from build123d import *

# Parameters (mm, degrees)
F1_DEPTH = 40.2336
F0_R     = 10.16
F2_DEPTH = 15.7734
F3_R     = 3.302


# Not quite as in the source:
# - a feature names something its author has since deleted; it is built from what else it names


with BuildPart() as f1:
    # F0 (on Top) → F1 (new body)
    with BuildSketch(Plane.XY):
        with BuildLine():
            ThreePointArc((-48.9323529412, -28.1265414802), (-32.0589754437, -18.3362616868), (-25.4, 0))
            ThreePointArc((-25.4, 0), (-32.0589754437, 18.3362616868), (-48.9323529412, 28.1265414802))
            ThreePointArc((-48.9323529412, 28.1265414802), (-82.55, 0), (-48.9323529412, -28.1265414802))
        make_face()
        with BuildLine():
            ThreePointArc((-40.5272351207, -4.826), (-68.2625, 0), (-40.5272351207, 4.826))
            Line((-40.5272351207, 4.826), (-34.1772351207, 4.826))
            Line((-34.1772351207, 4.826), (-34.1772351207, -4.826))
            Line((-34.1772351207, -4.826), (-40.5272351207, -4.826))
        make_face(mode=Mode.SUBTRACT)
    extrude(amount=F1_DEPTH)

    # F0 (on Top) → F2 (join)
    with BuildSketch(Plane.XY):
        with BuildLine():
            ThreePointArc((-48.9323529412, 28.1265414802), (-32.0589754437, 18.3362616868), (-25.4, 0))
            ThreePointArc((-25.4, 0), (-32.0589754437, -18.3362616868), (-48.9323529412, -28.1265414802))
            Line((-48.9323529412, -28.1265414802), (3.3617647059, -18.7510276535))
            ThreePointArc((3.3617647059, -18.7510276535), (-19.05, 0), (3.3617647059, 18.7510276535))
            Line((3.3617647059, 18.7510276535), (-48.9323529412, 28.1265414802))
        make_face()
        with BuildLine():
            ThreePointArc((19.05, 0), (14.6106830375, 12.2241744579), (3.3617647059, 18.7510276535))
            ThreePointArc((3.3617647059, 18.7510276535), (-19.05, 0), (3.3617647059, -18.7510276535))
            ThreePointArc((3.3617647059, -18.7510276535), (14.6106830375, -12.2241744579), (19.05, 0))
        make_face()
        Circle(F0_R, mode=Mode.SUBTRACT)
    extrude(amount=F2_DEPTH)

    # F3
    f3_edges = [f1.edges().sort_by_distance(p)[0] for p in [
        (-59.017647, 28.126541, 40.2336),
    ]]
    fillet(f3_edges, radius=F3_R)


solid = f1.part
Geometry: final body of the model. Coordinates: model frame, mm. A direction names the side the tool comes from. Give positions to 0.01 mm unless a question says otherwise; leave off trailing zeros. Order: outer loops, then holes, each group sorted by start corner. A loop starts at its lowest first (then second) coordinate and runs counter-clockwise, first axis right, second up. Notation, with made-up numbers: (67, 35) -> (106, 35) arc R21 ccw to (106, 58) -> close; hole circle Ø3 at (36.5, 1). An arc over 180 degrees is marked (long way). Write each question's results on one line, items separated by ' | '.
1) Draft query along Y for faces 1 (the face through (-22.419, 23.373, 7.776)), 2 (the face through (-37, -4.826, 20)), 3 (the face through (-23.151, -23.504, 7.776)). Return one class per face: released by +Y, released by -Y, zero draft, split by the parting line, or undercut.
Geometry says:
face 1: released by +Y | face 2: undercut | face 3: released by -Y
2) Set-up query: faces 4 (the face through (-32, 0, 0)), 5 (the face through (-37, 4.826, 20)). Return all of +Z, -Z, +X, -X, +Y, -Y with unobstructed straight access to the full face (end or side cutting, diameter ignored); none if empty.
Geometry says:
face 4: -Z, +X, -X, +Y, -Y | face 5: +Z, -Z
3) First-contact query: pin 1 Ø5 at (x, z) = (-38, 14.5) entering from +Y; pin 2 Ø7.5 at (y, z) = (-0.5, 25.5) entering from -X; pin 3 Ø1 at (x, y) = (-20, -6) entering from +Z. Flat tips, straight axial feed; report the tip coordinate or a pass-through.
Geometry says:
pin 1: stops at y = 26.61 | pin 2: stops at x = -82.55 | pin 3: stops at z = 15.77
4) Cut plane D-D (z = 38.5). Output: boundary loops of the cut face in (x, y) (1 decimal).
Geometry says:
outline: circle Ø56.4 at (-54, 0); hole (-40.5, -4.8) -> (-34.2, -4.8) -> (-34.2, 4.8) -> (-40.5, 4.8) arc R14.3 ccw (long way) to start
5) Cut plane C-C (y = -2.5). Give the number of separate pieces and of enclosed holes in the cut face, and give its area (3 significant figures).
Geometry says:
separate pieces: 3 | enclosed holes: 0 | area: 1,310 mm²
6) Cut plane A-A (x = 0). Output: boundary loops of the cut face in (y, z).
Geometry says:
outline: (-19.35, 0) -> (-10.16, 0) -> (-10.16, 15.77) -> (-19.35, 15.77) -> close; (10.16, 0) -> (19.35, 0) -> (19.35, 15.77) -> (10.16, 15.77) -> close
7) Line query: line 1 along X through (y, z) = (0, 30); line 2 along Z through (x, y) = (-16.5, -5); line 3 along X through (y, z) = (2, 34). Output: solid intervals per line, ascending.
Geometry says:
line 1: x = -82.55 to -68.26, -34.18 to -25.4 | line 2: z = 0 to 15.77 | line 3: x = -82.48 to -68.12, -34.18 to -25.47
